```python
from build123d import *

# Parameters (mm, degrees)
F1_DEPTH  = 38.1
F2_W      = 38.1
F2_H      = 38.1
F2_H_2    = 482.6
F3_DEPTH  = 3.175
F4_W      = 38.1
F4_H      = 38.1
F4_H_2    = 482.6
F5_DEPTH  = 3.175
F8_DEPTH  = 38.1
F9_DEPTH  = 38.1
F10_W     = 37.9836630458
F10_H     = 38.1
F11_DEPTH = 3.302
F12_DEPTH = 3.302


with BuildPart() as f1:
    # F0 (on Front) → F1 (new body)
    with BuildSketch(Plane.XZ):
        with BuildLine():
            Line((190.5, 0), (186.69, 37.9090213538))
            ThreePointArc((186.69, 37.9090213538), (166.9901958546, 91.6761936843), (132.2020589855, 137.16))
            Line((132.2020589855, 137.16), (102.2635224311, 160.72467757))
            ThreePointArc((102.2635224311, 160.72467757), (0, 190.5), (-102.2635224311, 160.72467757))
            Line((-102.2635224311, 160.72467757), (-132.2020589855, 137.16))
            ThreePointArc((-132.2020589855, 137.16), (-166.9901958546, 91.6761936843), (-186.69, 37.9090213538))
            Line((-186.69, 37.9090213538), (-190.5, 0))
            Line((-190.5, 0), (-184.15, 0))
            ThreePointArc((-184.15, 0), (0, 184.15), (184.15, 0))
            Line((184.15, 0), (190.5, 0))
        make_face()
    extrude(amount=F1_DEPTH)

    # F2 (on face) → F3 (join)
    with BuildSketch(Plane(origin=(-117.2327907083, 0, 148.942338785), x_dir=(0.785788361, 0, 0.6184954743), z_dir=(-0.6184954743, 0, 0.785788361))):
        with Locations((0, -19.05)):
            Rectangle(F2_W, F2_H)
        with Locations((0, 241.3)):
            Rectangle(F2_W, F2_H_2)
    extrude(amount=F3_DEPTH)

    # F4 (on face) → F5 (join)
    with BuildSketch(Plane(origin=(117.2327907083, 0, 148.942338785), x_dir=(0.785788361, 0, -0.6184954743), z_dir=(0.6184954743, 0, 0.785788361))):
        with Locations((0, -19.05)):
            Rectangle(F4_W, F4_H)
        with Locations((0, 241.3)):
            Rectangle(F4_W, F4_H_2)
    extrude(amount=F5_DEPTH)

    # F7 (on face) → F8 (join)
    with BuildSketch(Plane(origin=(0, 482.6, 0), x_dir=(-1, 0, 0), z_dir=(0, 1, 0))):
        with BuildLine():
            Line((130.004232963, 138.0423993869), (102.2635224311, 160.72467757))
            Line((102.2635224311, 160.72467757), (59.6745645386, 168.5625927845))
            ThreePointArc((59.6745645386, 168.5625927845), (96.0592635131, 156.1135098671), (130.004232963, 138.0423993869))
        make_face()
    extrude(amount=F8_DEPTH)



with BuildPart() as f9:
    # F6 (on face) → F9 (new body)
    with BuildSketch(Plane(origin=(0, 482.6, 0), x_dir=(-1, 0, 0), z_dir=(0, 1, 0))):
        with BuildLine():
            Line((236.22, -65.3515389739), (241.3, -65.3515389739))
            ThreePointArc((241.3, -65.3515389739), (160.6830293096, 114.6669436658), (-27.3005312217, 174.3991043934))
            Line((-27.3005312217, 174.3991043934), (-59.1095722207, 168.5966357826))
            ThreePointArc((-59.1095722207, 168.5966357826), (-96.7518090552, 155.7022496038), (-131.7632866386, 136.7972337016))
            ThreePointArc((-131.7632866386, 136.7972337016), (-212.1558048533, 49.607603625), (-241.3, -65.3515389739))
            Line((-241.3, -65.3515389739), (-236.22, -65.3515389739))
            ThreePointArc((-236.22, -65.3515389739), (0, 170.8684610261), (236.22, -65.3515389739))
        make_face()
        with BuildLine():
            ThreePointArc((-131.7632866386, 136.7972337016), (-96.7518090552, 155.7022496038), (-59.1095722207, 168.5966357826))
            Line((-59.1095722207, 168.5966357826), (-102.2635224311, 160.72467757))
            Line((-102.2635224311, 160.72467757), (-131.7632866386, 136.7972337016))
        make_face()
    extrude(amount=F9_DEPTH)


with BuildPart() as f1_1:
    add(f1.part)

    add(f9.part)  # F11 merges F9
    # F10 (on face) → F11 (join)
    with BuildSketch(Plane(origin=(119.2135098748, 0, 146.9764363882), x_dir=(0.7766434789, 0, -0.6299403994), z_dir=(0.6299403994, 0, 0.7766434789))):
        with Locations((-2.8328382326, 501.65)):
            Rectangle(F10_W, F10_H)
    extrude(amount=F11_DEPTH)

    # F12 (add): a face of the model
    f12_faces = [f1_1.faces().sort_by_distance(p)[0] for p in [
        (-116.133877697, 501.65, 149.3835384785),
    ]]
    extrude(f12_faces, amount=F12_DEPTH)


solid = f1_1.part
```
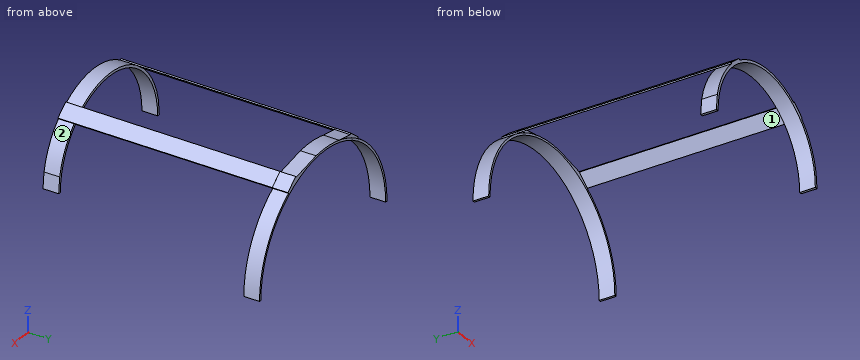
Model file for the job. Use its own axes, mm. Face numbers are marked on the shaded views. Round coordinates to 2 decimals unless told otherwise and drop trailing zeros. Write each loop counter-clockwise with the first axis right and the second up, starting at its lowest first coordinate (ties: lowest second). Pieces come first, ordered by that corner, then holes. Notation, with made-up numbers: (46, 33) - (60, 33) arc R30 cw to (60, 65) - close; hole circle Ø1 at (58, 68). An arc over 180 degrees is marked (long way). One line per item, written item: value.
(1) Drop flat-ended pins along their axis: P1, Ø2, axis at x = -103.5, z = 162.5, coming from the +Y side; P2, Ø7, axis at x = 188, y = -10.5, coming from the -Z side; P3, Ø15.5, axis at x = -82.5, z = 154, coming from the -Y side; P4, Ø4, axis at y = 32.5, z = 146.5, coming from the +X side. Give the stop position or say it passes through.
Values follow:
P1: stops at y = 520.7
P2: stops at z = 0
P3: stops at y = 482.6
P4: stops at x = 128.01
(2) Wall check: probe 1 along X at (y, z) = (463.5, 157); probe 2 along Z at (x, y) = (-111, 175.5); probe 3 along X at (y, z) = (383.5, 151.5). Give the ranges that are in metal, low to high.
Values follow:
probe 1: x = -112.13 to -107, 107 to 112.13
probe 2: z = 153.85 to 157.89
probe 3: x = -119.12 to -113.98, 113.98 to 119.12
(3) Two-plate mould, pull along Y, no slides. Class the marked faces 1 and 2: pulls with the +Y half, pulls with the -Y half, needs draft (parallel to the pull), parting line crosses it, or undercut.
Values follow:
face 1: undercut
face 2: needs draft
(4) Cut at B-B, the plane x = 0. Give the cut face in (y, z).
Values follow:
outline: (-38.1, 184.15) - (0, 184.15) - (0, 190.5) - (-38.1, 190.5) - close; (482.6, 170.87) - (520.7, 170.87) - (520.7, 175.95) - (482.6, 175.95) - close
(5) Cut at C-C, the plane z = 86. Give the cut face in (x, y).
Values follow:
outline: (-187.93, 482.6) - (-181.36, 482.6) - (-181.36, 520.7) - (-187.93, 520.7) - close; (-169.98, -38.1) - (-162.83, -38.1) - (-162.83, 0) - (-169.98, 0) - close; (162.83, -38.1) - (169.98, -38.1) - (169.98, 0) - (162.83, 0) - close; (181.36, 482.6) - (187.93, 482.6) - (187.93, 520.7) - (181.36, 520.7) - close
(6) Cut at D-D, the plane z = 46. Give the cut face in (x, y).
Values follow:
outline: (-214.07, 482.6) - (-208.33, 482.6) - (-208.33, 520.7) - (-214.07, 520.7) - close; (-184.86, -38.1) - (-178.31, -38.1) - (-178.31, 0) - (-184.86, 0) - close; (178.31, -38.1) - (184.86, -38.1) - (184.86, 0) - (178.31, 0) - close; (208.33, 482.6) - (214.07, 482.6) - (214.07, 520.7) - (208.33, 520.7) - close
(7) Cut at A-A, the plane y = 452. Give the cut face in (x, z), plus the area to 3 significant figures.
Values follow:
outline: (-134.17, 139.65) - (-132.2, 137.16) - (-102.26, 160.72) - (-104.23, 163.22) - close; (102.26, 160.72) - (132.2, 137.16) - (134.17, 139.65) - (104.23, 163.22) - close
area: 242 mm²
